Read the model definition and answer for the solid it produces. Units are mm, in the model's axes. A direction names the side the tool comes from. Coordinates: 2 decimals unless noted, no trailing zeros. Write each loop counter-clockwise with the first axis right and the second up, starting at its lowest first coordinate (ties: lowest second). Pieces come first, ordered by that corner, then holes. Notation, with made-up numbers: (63.5, -2.75) -> (110.5, -2.75) arc R34 ccw to (110.5, 32.25) -> close; hole circle Ø9 at (-33.5, 39.5). An arc over 180 degrees is marked (long way). Use CSV: the item, a comma, the result in double quotes. Start each with the question number.
from build123d import *

# Parameters (mm, degrees)
SKETCH1_W                = 92
SKETCH1_H                = 12
BOSS_EXTRUDE1_DEPTH      = 3
FILLET1_R                = 4
CUT_EXTRUDE1_DEPTH       = 3
SKETCH3_R                = 5
BOSS_EXTRUDE2_DEPTH      = 3
BOSS_EXTRUDE2_DEPTH_BACK = 3


with BuildPart() as part:
    # Sketch1 → Boss-Extrude1 (new body)
    with BuildSketch(Plane.XY):
        Rectangle(SKETCH1_W, SKETCH1_H)
    extrude(amount=BOSS_EXTRUDE1_DEPTH)

    # Fillet1
    fillet1_edges = [part.edges().sort_by_distance(p)[0] for p in [
        (-46, -6, 1.5),
        (-46, 6, 1.5),
    ]]
    fillet(fillet1_edges, radius=FILLET1_R)

    # Sketch2 → Cut-Extrude1 (cut)
    with BuildSketch(Plane.XY.offset(3)):
        with BuildLine():
            Line((-43, 2), (-43, -2))
            ThreePointArc((-43, -2), (-42.707106781, -2.707106781), (-42, -3))
            Line((-42, -3), (43, -3))
            Line((43, -3), (43, 3))
            Line((43, 3), (-42, 3))
            ThreePointArc((-42, 3), (-42.707106781, 2.707106781), (-43, 2))
        make_face()
    extrude(amount=-CUT_EXTRUDE1_DEPTH, mode=Mode.SUBTRACT)

    # Sketch3 → Boss-Extrude2 (add, two sides)
    with BuildSketch(Plane.XY.offset(3)) as boss_extrude2_sk:
        with Locations((-40, 0)):
            Circle(SKETCH3_R)
    extrude(amount=BOSS_EXTRUDE2_DEPTH)
    extrude(boss_extrude2_sk.sketch, amount=-BOSS_EXTRUDE2_DEPTH_BACK)


solid = part.part
1) Find the intervals of material crossed by line 1 along Y through (x, z) = (15, 2.95); line 2 along Z through (x, y) = (9, 4.25); line 3 along X through (y, z) = (-1.5, 2.6), in increasing order.
2) The mould has two halves that part along X. Classify faces 3 (the face through (46, 0, 1)), 4 (the face through (-1, -4, 3)), 5 (the face through (3, -3, 2)): pulls with the +X half, pulls with the -X half, needs draft (parallel to the pull), parting line crosses it, or undercut.
3) Section D-D, the plane y = -3.75 is taken. Give the vertices of the cut face in (x, z), plus the area to 3 significant figures.
4) Section A-A, the plane x = 1 is taken. Give the vertices of the cut face in (y, z).
5) Each of these flat-tipped pins is pushed along its axis until it touches: pin 1 (2 mm diameter, centred on x = -19.5, y = -3, fed in from +Z); pin 2 (2 mm diameter, centred on x = -18.5, y = 1, fed in from +Z). Where does it stop, or does it pass through?
6) Section B-B, the plane z = 1.05 is taken. Give the vertices of the cut face in (x, y).
7) Section C-C, the plane x = -40 is taken. Give the vertices of the cut face in (y, z), plus the area to 3 significant figures.
8) Which of the six approach directions +Z, -Z, +X, -X, +Y, -Y give full straight-line access (tool end or side, diameter ignored) to faces 1 (the face through (-44.859, 4.797, 1.521)), 2 (the face through (43, 0, 2))?
The answers:
1,line 1,"y = -6 to -3, 3 to 6"
1,line 2,"z = 0 to 3"
1,line 3,"x = -46 to -35.23, 43 to 46"
2,face 3,"pulls with the +X half"
2,face 4,"needs draft"
2,face 5,"undercut"
3,outline,"(-45.6, 0) -> (46, 0) -> (46, 3) -> (-36.69, 3) -> (-36.69, 6) -> (-43.31, 6) -> (-43.31, 3) -> (-45.6, 3) -> close"
3,area,"295 mm^2"
4,outline,"(-6, 0) -> (-3, 0) -> (-3, 3) -> (-6, 3) -> close; (3, 0) -> (6, 0) -> (6, 3) -> (3, 3) -> close"
5,pin 1,"stops at z = 3"
5,pin 2,"passes through"
6,outline,"(-46, -2) arc R4 ccw to (-42, -6) -> (46, -6) -> (46, 6) -> (-42, 6) arc R4 ccw to (-46, 2) -> close; hole (-36, -3) -> (43, -3) -> (43, 3) -> (-36, 3) arc R5 cw to start"
7,outline,"(-6, 0) -> (6, 0) -> (6, 3) -> (5, 3) -> (5, 6) -> (-5, 6) -> (-5, 3) -> (-6, 3) -> close"
7,area,"66.0 mm^2"
8,face 1,"+Z, -Z, -X, +Y"
8,face 2,"+Z, -Z"
